Source: CAD feature listing. Evaluate the final solid. Frame: model axes, mm. A direction names the side the tool comes from. Give positions to 0.01 mm unless a question says otherwise; leave off trailing zeros. Order: outer loops, then holes, each group sorted by start corner. A loop starts at its lowest first (then second) coordinate and runs counter-clockwise, first axis right, second up.
from build123d import *

# Parameters (mm, degrees)
SKETCH1_W                      = 158
SKETCH1_H                      = 199.5
BOSS_EXTRUDE1_DEPTH            = 6.35
BOSS_EXTRUDE2_DEPTH            = 12.7
CBORE_FOR_M4_SHCS1_D           = 4.5
CBORE_FOR_M4_SHCS1_DEPTH       = 6.35
CBORE_FOR_M4_SHCS1_CBORE_D     = 8
CBORE_FOR_M4_SHCS1_CBORE_DEPTH = 4
F_5_1_5_1_DIAMETER_HOLE1_D     = 5.1
F_5_1_5_1_DIAMETER_HOLE1_DEPTH = 6.35
FILLET2_R                      = 5
FILLET3_R                      = 5
F_5_0_5_DIAMETER_HOLE1_D       = 5
F_5_0_5_DIAMETER_HOLE1_DEPTH   = 6.35


with BuildPart() as part:
    # Sketch1 → Boss-Extrude1 (new body)
    with BuildSketch(Plane(origin=(0, 0, 0), x_dir=(1, 0, 0), z_dir=(0, 1, 0))):
        with Locations((79, -99.75)):
            Rectangle(SKETCH1_W, SKETCH1_H)
    extrude(amount=BOSS_EXTRUDE1_DEPTH)

    # Sketch3 → Boss-Extrude2 (add)
    with BuildSketch(Plane(origin=(0, 6.35, 0), x_dir=(1, 0, 0), z_dir=(0, 1, 0))):
        Polygon((158, -199.5), (158, 0), (153, 0), (153, -194.5), (0, -194.5), (0, -199.5), align=None)
    extrude(amount=BOSS_EXTRUDE2_DEPTH)

    # CBORE for M4 SHCS1
    with Locations(Plane(origin=(0, 6.35, 0), x_dir=(1, 0, 0), z_dir=(0, 1, 0))):
        with Locations((138, -55), (20, -179.5), (60, -179.5), (138, -130), (138, -105), (138, -30)):
            CounterBoreHole(CBORE_FOR_M4_SHCS1_D / 2, CBORE_FOR_M4_SHCS1_CBORE_D / 2, CBORE_FOR_M4_SHCS1_CBORE_DEPTH, depth=CBORE_FOR_M4_SHCS1_DEPTH)

    # Ø5.1 (5.1) Diameter Hole1
    with Locations(Plane(origin=(0, 6.35, 0), x_dir=(1, 0, 0), z_dir=(0, 1, 0))):
        with Locations((43, -40.38), (43, -122.25), (93, -122.25), (93, -40.38)):
            Hole(F_5_1_5_1_DIAMETER_HOLE1_D / 2, depth=F_5_1_5_1_DIAMETER_HOLE1_DEPTH)

    # Fillet2
    fillet2_edges = [part.edges().sort_by_distance(p)[0] for p in [
        (158, 9.525, 199.5),
    ]]
    fillet(fillet2_edges, radius=FILLET2_R)

    # Fillet3
    fillet3_edges = [part.edges().sort_by_distance(p)[0] for p in [
        (153, 12.7, 194.5),
    ]]
    fillet(fillet3_edges, radius=FILLET3_R)

    # Ø5.0 (5) Diameter Hole1
    with Locations(Plane(origin=(0, 6.35, 0), x_dir=(1, 0, 0), z_dir=(0, 1, 0))):
        with Locations((31, -159.5), (143, -159.5)):
            Hole(F_5_0_5_DIAMETER_HOLE1_D / 2, depth=F_5_0_5_DIAMETER_HOLE1_DEPTH)


solid = part.part
(1) Section B-B, the plane z = 55. Return loops of the section in (x, y).
(2) Section D-D, the plane z = 113. Return loops of the section in (x, y).
(3) Draft query along X for faces 1 (the flat face through (75, 9, 199.5)), 2 (the cylindrical face through (135.92, 1.16, 30.86)), 3 (the cylindrical face through (151.57, 12.79, 193)), 4 (the cylindrical face through (31, 3, 157)). Return one class per face: +X half, -X half, draft (parallel to the pull), parting line (faces both ways), or undercut.
(4) Access query for faces 5 (the flat face through (140, 2.35, 107)), 6 (the cylindrical face through (60.488, 1.159, 181.696)), 7 (the flat face through (75, 6.35, 96)). Directions: +Z, -Z, +X, -X, +Y, -Y. A direction counts if a zero-diameter tool reaches every point of the face in a straight line with its end or side. Return the directions, or none.
(5) Section C-C, the plane x = 43. Return loops of the section in (y, z).
(6) Section A-A, the plane x = 20. Return loops of the section in (y, z).
(7) Line query: line 1 along X through (y, z) = (5, 40.38); line 2 along Z through (x, y) = (138, 3.3); line 3 along X through (y, z) = (0.95, 179.5). Output: solid intervals per line, ascending.
(8) Pin query (flat end, axial travel): pin 1 Ø2.5 at (x, z) = (136.5, 105.5) entering from +Y; pin 2 Ø6 at (y, z) = (14.5, 85.5) entering from -X; pin 3 Ø5 at (x, y) = (116.5, 14) entering from -Z. Return the tip coordinate at first contact, or that it passes through.
Checks:
1. outline: (0, 0) - (135.75, 0) - (135.75, 2.35) - (134, 2.35) - (134, 6.35) - (0, 6.35) - close; (140.25, 0) - (158, 0) - (158, 19.05) - (153, 19.05) - (153, 6.35) - (142, 6.35) - (142, 2.35) - (140.25, 2.35) - close
2. outline: (0, 0) - (158, 0) - (158, 19.05) - (153, 19.05) - (153, 6.35) - (0, 6.35) - close
3. face 1: draft
3. face 2: undercut
3. face 3: -X half
3. face 4: undercut
4. face 5: +Y
4. face 6: +Y, -Y
4. face 7: -Z, -X, +Y
5. outline: (0, 0) - (6.35, 0) - (6.35, 37.83) - (0, 37.83) - close; (0, 42.93) - (6.35, 42.93) - (6.35, 119.7) - (0, 119.7) - close; (0, 124.8) - (6.35, 124.8) - (6.35, 194.5) - (19.05, 194.5) - (19.05, 199.5) - (0, 199.5) - close
6. outline: (0, 0) - (6.35, 0) - (6.35, 175.5) - (2.35, 175.5) - (2.35, 177.25) - (0, 177.25) - close; (0, 181.75) - (2.35, 181.75) - (2.35, 183.5) - (6.35, 183.5) - (6.35, 194.5) - (19.05, 194.5) - (19.05, 199.5) - (0, 199.5) - close
7. line 1: x = 0 to 40.45, 45.55 to 90.45, 95.55 to 158
7. line 2: z = 0 to 26, 34 to 51, 59 to 101, 109 to 126, 134 to 199.5
7. line 3: x = 0 to 17.75, 22.25 to 57.75, 62.25 to 158
8. pin 1: stops at y = 2.35
8. pin 2: stops at x = 153
8. pin 3: stops at z = 194.5
